```python
from build123d import *

# Parameters (mm, degrees)
SKETCH1_W                   = 100
SKETCH1_H                   = 19
SKETCH1_W_2                 = 38
SKETCH1_H_2                 = 25
BOSS_EXTRUDE1_DEPTH         = 64
CUT_EXTRUDE1_DEPTH          = 13
CUT_EXTRUDE2_DEPTH          = 20
CUT_EXTRUDE3_DEPTH          = 101
TAP_DRILL_FOR_M6_TAP1_D     = 5
TAP_DRILL_FOR_M6_TAP1_DEPTH = 20
TAP_DRILL_FOR_M6_TAP1_TIP   = 1.502151548
SKETCH9_R                   = 5
CUT_EXTRUDE4_DEPTH          = 32


with BuildPart() as part:
    # Sketch1 → Boss-Extrude1 (new body)
    with BuildSketch(Plane.XY):
        with Locations((5.391120507, -14.601479915)):
            Rectangle(SKETCH1_W, SKETCH1_H)
        with Locations((36.391120507, 7.398520085)):
            Rectangle(SKETCH1_W_2, SKETCH1_H_2)
    extrude(amount=-BOSS_EXTRUDE1_DEPTH)

    # Sketch2 → Cut-Extrude1 (cut)
    with BuildSketch(Plane(origin=(0, 19.898520085, 0), x_dir=(1, 0, 0), z_dir=(0, 1, 0))):
        Polygon((55.391120507, 44), (55.391120507, 20), (17.391120507, 13), (17.391120507, 51), align=None)
    extrude(amount=-CUT_EXTRUDE1_DEPTH, mode=Mode.SUBTRACT)

    # Sketch3 → Cut-Extrude2 (cut, through all)
    with BuildSketch(Plane(origin=(0, -5.101479915, 0), x_dir=(1, 0, 0), z_dir=(0, 1, 0))):
        with BuildLine():
            Line((-23.608879493, 42), (-5.608879493, 42))
            ThreePointArc((-5.608879493, 42), (4.391120507, 32), (-5.608879493, 22))
            Line((-5.608879493, 22), (-23.608879493, 22))
            ThreePointArc((-23.608879493, 22), (-33.608879493, 32), (-23.608879493, 42))
        make_face()
    extrude(amount=-CUT_EXTRUDE2_DEPTH, mode=Mode.SUBTRACT)

    # Sketch5 → Cut-Extrude3 (cut, through all)
    with BuildSketch(Plane.ZY.offset(44.608879493)):
        Polygon((-14.043777718, -15.101479915), (-7, -15.101479915), (-7, -24.101479915), (-57, -24.101479915), (-57, -15.101479915), (-52.287609929, -15.101479915), align=None)
    extrude(amount=-CUT_EXTRUDE3_DEPTH, mode=Mode.SUBTRACT)

    # Tap Drill for M6 Tap1
    with Locations(Plane(origin=(0, 19.898520085, 0), x_dir=(1, 0, 0), z_dir=(0, 1, 0))):
        with Locations((42.391120507, 54), (42.391120507, 10)):
            Hole(TAP_DRILL_FOR_M6_TAP1_D / 2, depth=TAP_DRILL_FOR_M6_TAP1_DEPTH)
            with Locations((0, 0, -(TAP_DRILL_FOR_M6_TAP1_DEPTH + TAP_DRILL_FOR_M6_TAP1_TIP / 2))):  # 118° drill point
                Cone(0, TAP_DRILL_FOR_M6_TAP1_D / 2, TAP_DRILL_FOR_M6_TAP1_TIP, mode=Mode.SUBTRACT)

    # Sketch9 → Cut-Extrude4 (cut, through all)
    with BuildSketch(Plane(origin=(0, 6.898520085, 0), x_dir=(1, 0, 0), z_dir=(0, 1, 0))):
        with Locations((36.391120507, 32)):
            Circle(SKETCH9_R)
    extrude(amount=-CUT_EXTRUDE4_DEPTH, mode=Mode.SUBTRACT)


solid = part.part
```
Geometry: final body of the model. Coordinates: model frame, mm. A direction names the side the tool comes from. Coordinates: 2 decimals unless noted, no trailing zeros. Write each loop counter-clockwise with the first axis right and the second up, starting at its lowest first coordinate (ties: lowest second). Pieces come first, ordered by that corner, then holes. Notation, with made-up numbers: M -11.75,-21 L 39.25,-21 A18 ccw 39.25,-1 Z; hole C 63.25,-19 d1. An arc over 180 degrees is marked long. Use CSV: the item, a comma, the result in double quotes. Start each with the question number.
1. Cut plane B-B on z = -32. Return the cut outline in (x, y), plus the area to 3 significant figures.
2. Cut plane C-C on y = 3. Return the cut outline in (x, z).
3. First-contact query: P1, Ø16, axis at x = 36.39, z = -32, coming from the -Y side; P2, Ø6, axis at x = -33, z = -52, coming from the +Y side. Flat tips, straight axial feed; report the tip coordinate or a pass-through.
4. Reachability of faces 5 (the face through (5, -15.101, -32)), 6 (the face through (36.66, 13.49, -16.55)), 7 (the face through (-14, -10, -22)), 8 (the face through (17.391, 4, -32)) from +Z, -Z, +X, -X, +Y, -Y: full face, straight path, thin tool, end or side. Return the list, or none.
5. Ray query, probe 1 along X at (y, z) = (-6, -32); probe 2 along X at (y, z) = (14, -10); probe 3 along Z at (x, y) = (-13, -11). Return the intervals inside material, ascending.
6. Mould query, pull axis X, two halves, no side actions, for faces 1 (the face through (42.792, -1.343, -53.834)), 2 (the face through (55.391, -2, -32)), 3 (the face through (16, -7, 0)), 4 (the face through (-44.609, -13, -32)). Classes: pulls with the +X half, pulls with the -X half, needs draft (parallel to the pull), parting line crosses it, or undercut.
7. Cut plane A-A on y = 16. Return the cut outline in (x, z).
8. Cut plane D-D on x = 47. Return the cut outline in (y, z), plus the area to 3 significant figures.
Entries:
1,outline,"M -44.61,-15.1 L -33.61,-15.1 L -33.61,-5.1 L -44.61,-5.1 Z; M 4.39,-15.1 L 31.39,-15.1 L 31.39,6.9 L 17.39,6.9 L 17.39,-5.1 L 4.39,-5.1 Z; M 41.39,-15.1 L 55.39,-15.1 L 55.39,6.9 L 41.39,6.9 Z"
1,area,"856 mm²"
2,outline,"M 17.39,-64 L 55.39,-64 L 55.39,0 L 17.39,0 Z; hole C 36.39,-32 d10; hole C 42.39,-54 d5; hole C 42.39,-10 d5"
3,P1,"y = -15.1"
3,P2,"y = -5.1"
4,face 5,"+X, -X, -Y"
4,face 6,"-X, +Y"
4,face 7,"+Y, -Y"
4,face 8,"+Z, -Z, -X, +Y"
5,probe 1,"-44.61 to -33.61, 4.39 to 31.39, 41.39 to 55.39"
5,probe 2,"17.39 to 39.89, 44.89 to 55.39"
5,probe 3,"-64 to -42, -22 to 0"
6,face 1,"undercut"
6,face 2,"pulls with the +X half"
6,face 3,"needs draft"
6,face 4,"pulls with the -X half"
7,outline,"M 17.39,-64 L 55.39,-64 L 55.39,-44 L 17.39,-51 Z; M 17.39,-13 L 55.39,-20 L 55.39,0 L 17.39,0 Z; hole C 42.39,-54 d5; hole C 42.39,-10 d5"
8,outline,"M -24.1,-64 L 19.9,-64 L 19.9,-45.55 L 6.9,-45.55 L 6.9,-18.45 L 19.9,-18.45 L 19.9,0 L -24.1,0 L -24.1,-7 L -15.1,-7 L -15.1,-57 L -24.1,-57 Z"
8,area,"2,010 mm²"
